Could you check a few things on this model? Use its own coordinates, in mm. A direction names the side the tool comes from. Coordinates: 2 decimals unless noted, no trailing zeros. Write each loop counter-clockwise with the first axis right and the second up, starting at its lowest first coordinate (ties: lowest second). Pieces come first, ordered by that corner, then holes.
```python
from build123d import *

# Parameters (mm, degrees)
BOSS_EXTRUDE1_DEPTH              = 36
SKETCH2_R                        = 7.5
BOSS_EXTRUDE2_DEPTH              = 4
SKETCH3_R                        = 15
SKETCH3_R_2                      = 7.5
BOSS_EXTRUDE3_DEPTH              = 5
FILLET2_R                        = 15
RIB1_REACH                       = 83.598
SKETCH4_WALL_W                   = 212.903642704
SKETCH4_WALL_H                   = 10
FILLET3_R                        = 12
M12X1_5_TAPPED_HOLE1_D           = 10.5
M12X1_5_TAPPED_HOLE1_CSINK_D     = 12.05
M12X1_5_TAPPED_HOLE1_CSINK_ANGLE = 90


with BuildPart() as part:
    # Sketch1 → Boss-Extrude1 (new, symmetric)
    with BuildSketch(Plane(origin=(0, 0, 0), x_dir=(0, 0, -1), z_dir=(1, 0, 0))):
        Polygon((-17.5, 1), (-17.5, -5), (17.5, -5), (17.5, 5), (-12.5, 5), (-12.5, 1), align=None)
    extrude(amount=BOSS_EXTRUDE1_DEPTH, both=True)

    # Sketch2 → Boss-Extrude2 (add, symmetric)
    with BuildSketch(Plane.XY.offset(12.5)):
        with BuildLine():
            ThreePointArc((15, 55), (0, 70), (-15, 55))
            Line((-15, 55), (-15, 5))
            Line((-15, 5), (15, 5))
            Line((15, 5), (15, 55))
        make_face()
        with Locations((0, 55)):
            Circle(SKETCH2_R, mode=Mode.SUBTRACT)
    extrude(amount=BOSS_EXTRUDE2_DEPTH, both=True)

    # Sketch3 → Boss-Extrude3 (add)
    with BuildSketch(Plane.XY.offset(16.5)):
        with Locations((0, 55)):
            Circle(SKETCH3_R)
        with Locations((0, 55)):
            Circle(SKETCH3_R_2, mode=Mode.SUBTRACT)
    extrude(amount=BOSS_EXTRUDE3_DEPTH)

    # Fillet2
    fillet2_edges = [part.edges().sort_by_distance(p)[0] for p in [
        (-15, 5, 10.5),
        (15, 5, 10.5),
    ]]
    fillet(fillet2_edges, radius=FILLET2_R)

    # Sketch4 wall → Rib1 (add, up to next)
    with BuildSketch(Plane(origin=(0, 25, -4.5), x_dir=(0, 0.838443616301, 0.544988350595), z_dir=(0, -0.544988350595, 0.838443616301)), mode=Mode.PRIVATE) as rib1_sk1:
        Rectangle(SKETCH4_WALL_W, SKETCH4_WALL_H)
    rib1_tool1 = extrude(rib1_sk1.sketch, amount=RIB1_REACH, mode=Mode.PRIVATE) - part.part
    add(rib1_tool1.solids().sort_by_distance((0, 25, -4.5))[0])

    # Fillet3
    fillet3_edges = [part.edges().sort_by_distance(p)[0] for p in [
        (36, 0, -17.5),
        (-36, 0, -17.5),
    ]]
    fillet(fillet3_edges, radius=FILLET3_R)

    # M12x1.5 Tapped Hole1 (through all)
    with Locations(Plane(origin=(0, 5, 0), x_dir=(1, 0, 0), z_dir=(0, 1, 0))):
        with Locations((24, 5.5), (-24, 5.5)):
            CounterSinkHole(M12X1_5_TAPPED_HOLE1_D / 2, M12X1_5_TAPPED_HOLE1_CSINK_D / 2, counter_sink_angle=M12X1_5_TAPPED_HOLE1_CSINK_ANGLE)


solid = part.part
```
Item 1: Which directions (+Z, -Z, +X, -X, +Y, -Y) give clear straight access to the entire face, cutting with the end or side of a thin tool? Please do faces 5 (the flat face through (-15, 36, 13)), 6 (the flat face through (6, 38, 8.5)), 7 (the flat face through (15, 35, 13)), 8 (the flat face through (-17, 5, -3)), 9 (the flat face through (-0.07, 24.72, -4.68)).
Item 2: Will these pins go through, and if not, where does the flat tip stop? pin 1 Ø4 at (x, y) = (16, 17.5) entering from +Z; pin 2 Ø9 at (y, z) = (39.5, 11.5) entering from +X; pin 3 Ø21 at (x, y) = (12.5, 9) entering from +Z.
Item 3: I want a section at A-A, the plane z = 15.5. List the corners of the cut face in (x, y) for me, then the cut area to 3 significant figures.
Item 4: If I drill on line 1 along Y through (x, z) = (0, 14); line 2 along Z through (x, y) = (-24, 0); line 3 along X through (y, z) = (25, 15), over which ranges is the centre line in solid material (lowest first)?
Item 5: I want a section at C-C, the plane y = 50. List the corners of the cut face in (x, z) for me, then the cut area to 3 significant figures.
Item 6: If we mould it in two halves opening along Y, with no side actions, what happens to faces 1 (the flat face through (0, 5, 15)), 2 (the cylindrical face through (19.28, 9.51, 10.47)), 3 (the cylindrical face through (-1.63, 47.68, 14.91)), 4 (the flat face through (1, -2, 17.5))? For each: released by +Y, released by -Y, zero draft, split by the parting line, or undercut.
Item 7: I want a section at B-B, the plane x = 0. List the corners of the cut face in (y, z) for me, then the cut area to 4 significant figures.
Item 8: I want a section at D-D, the plane z = 3. List the corners of the cut face in (x, y) for me, then the cut area to 3 significant figures.
Taken from the geometry:
1. face 5: +Z, -X, +Y
1. face 6: -Z, +Y
1. face 7: +Z, +X, +Y
1. face 8: -Z, -X, +Y
1. face 9: -Z, +X, -X, +Y
2. pin 1: stops at z = 16.5
2. pin 2: stops at x = 15
2. pin 3: stops at z = 17.5
3. outline: (-36, -5) - (36, -5) - (36, 1) - (-36, 1) - close; (-15, 5) - (15, 5) - (15, 55) arc R15 ccw to (-15, 55) - close; hole circle Ø15 at (0, 55)
3. area: 2,110 mm2
4. line 1: y = -5 to 1, 5 to 47.5, 62.5 to 70
4. line 2: z = -17.5 to -10.75, -0.25 to 17.5
4. line 3: x = -15 to 15
5. outline: (-15, 8.5) - (-5.59, 8.5) - (-5.59, 21.5) - (-14.14, 21.5) - (-14.14, 16.5) - (-15, 16.5) - close; (5.59, 8.5) - (15, 8.5) - (15, 16.5) - (14.14, 16.5) - (14.14, 21.5) - (5.59, 21.5) - close
5. area: 236 mm2
6. face 1: undercut
6. face 2: released by +Y
6. face 3: undercut
6. face 4: zero draft
7. outline: (-5, -17.5) - (5, -17.5) - (45, 8.5) - (47.5, 8.5) - (47.5, 21.5) - (40, 21.5) - (40, 16.5) - (5, 16.5) - (5, 12.5) - (1, 12.5) - (1, 17.5) - (-5, 17.5) - close; (62.5, 8.5) - (70, 8.5) - (70, 21.5) - (62.5, 21.5) - close
7. area: 1,325 mm2
8. outline: (-36, -5) - (36, -5) - (36, 5) - (5, 5) - (5, 36.54) - (-5, 36.54) - (-5, 5) - (-36, 5) - close
8. area: 1,040 mm2
